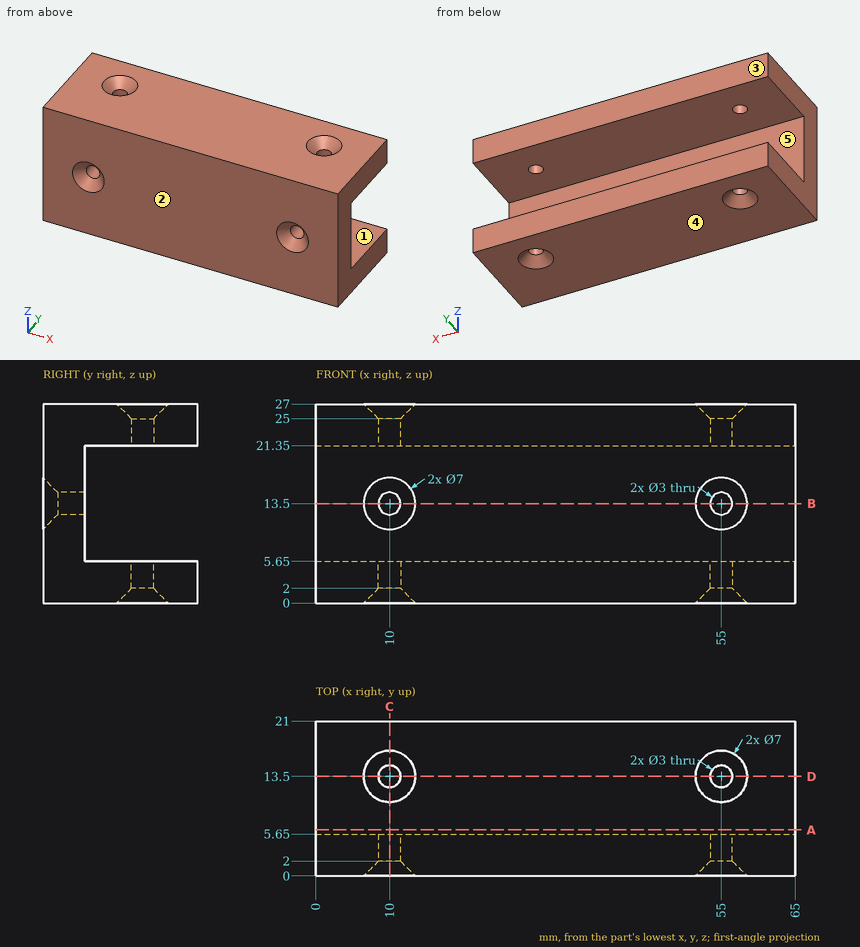
The drawing under review shows one solid part. Ordinate dimensions are in mm from its lowest x, y, z. A direction names the side the tool comes from. Give positions to 0.01 mm unless a question says otherwise; leave off trailing zeros. Order: outer loops, then holes, each group sorted by start corner. A loop starts at its lowest first (then second) coordinate and runs counter-clockwise, first axis right, second up. Notation, with made-up numbers: (57.5, 80.5) -> (107.5, 80.5) arc R25 ccw to (107.5, 92.5) -> close; hole circle Ø1 at (60, -14). An arc over 180 degrees is marked (long way). Write item = value, one per line. Start each with the question number.
(1) We need section B-B on z = 13.5. Write out the cut boundary in (x, y).
(2) Mouldability with a two-part tool opening along Z and no side actions: class the marked faces 3, 4 and 5 as +Z half, -Z half, draft (parallel to the pull), parting line (faces both ways), or undercut.
(3) We need section D-D on y = 13.5. State how many separate pieces and enclosed holes the cut face has, plus the area to 3 significant figures.
(4) We need section A-A on y = 6.25. Write out the cut boundary in (x, z).
(5) For pin 1 (2.5 mm diameter, centred on x = 55, y = 13.5, fed in from +Z); pin 2 (3 mm diameter, centred on x = 12.5, z = 9.5, fed in from -Y); pin 3 (5 mm diameter, centred on x = 55, y = 13.5, fed in from +Z); pin 4 (3.5 mm diameter, centred on x = 10, z = 13.5, fed in from +Y), all flat-tipped, find the tip position at first contact; note any pin that passes through.
(6) For the marked faces 1 and 2, list the 3-axis set-ups (+Z, -Z, +X, -X, +Y, -Y) from which the entire face can be reached by the end or side of a thin tool; tool diameter is ignored.
(7) To check wall thickness, follow line 1 along X through (y, z) = (13.5, 23.95); line 2 along Y through (x, z) = (55, 3.45); line 3 along Z through (x, y) = (55, 4.65). State the ranges of each line that lie inside material, in increasing order.
(8) We need section C-C on x = 10. Write out the cut boundary in (y, z).
Numbers:
q1.outline = (0, 0) -> (6.5, 0) -> (8.5, 2) -> (8.5, 5.65) -> (0, 5.65) -> close; (11.5, 2) -> (13.5, 0) -> (51.5, 0) -> (53.5, 2) -> (53.5, 5.65) -> (11.5, 5.65) -> close; (56.5, 2) -> (58.5, 0) -> (65, 0) -> (65, 5.65) -> (56.5, 5.65) -> close
q2.face_3 = draft
q2.face_4 = -Z half
q2.face_5 = undercut
q3.separate_pieces = 6
q3.enclosed_holes = 0
q3.area = 651 mm^2
q4.outline = (0, 0) -> (65, 0) -> (65, 5.65) -> (0, 5.65) -> close; (0, 21.35) -> (65, 21.35) -> (65, 27) -> (0, 27) -> close
q5.pin_1 = through
q5.pin_2 = 0
q5.pin_3 = 26
q5.pin_4 = 5.65
q6.face_1 = +X, -X, +Y
q6.face_2 = +Z, -Z, +X, -X, -Y
q7.line_1 = 0 to 8.5, 11.5 to 53.5, 56.5 to 65
q7.line_2 = 0 to 12, 15 to 21
q7.line_3 = 0 to 12, 15 to 27
q8.outline = (0, 0) -> (10, 0) -> (12, 2) -> (12, 5.65) -> (5.65, 5.65) -> (5.65, 12) -> (2, 12) -> (0, 10) -> close; (0, 17) -> (2, 15) -> (5.65, 15) -> (5.65, 21.35) -> (12, 21.35) -> (12, 25) -> (10, 27) -> (0, 27) -> close; (15, 2) -> (17, 0) -> (21, 0) -> (21, 5.65) -> (15, 5.65) -> close; (15, 21.35) -> (21, 21.35) -> (21, 27) -> (17, 27) -> (15, 25) -> close
